```python
from build123d import *

# Parameters (mm, degrees)
BOSS_EXTRUDE1_DEPTH = 5
SKETCH2_W           = 30
SKETCH2_H           = 5
CUT_EXTRUDE1_DEPTH  = 5


with BuildPart() as part:
    # Sketch1 → Boss-Extrude1 (new body)
    with BuildSketch(Plane.XY):
        Polygon((-75.513214474, 35), (-60.513214474, 35), (-60.513214474, 40), (-40.513214474, 40), (-40.513214474, 35), (-25.513214474, 35), (-25.513214474, 40), (-5.513214474, 40), (-5.513214474, 35), (9.486785526, 35), (9.486785526, 40), (29.486785526, 40), (29.486785526, 35), (44.486785526, 35), (44.486785526, 40), (64.486785526, 40), (64.486785526, 35), (79.486785526, 35), (79.486785526, 25), (84.486785526, 25), (84.486785526, 5), (79.486785526, 5), (79.486785526, -5), (84.486785526, -5), (84.486785526, -25), (79.486785526, -25), (79.486785526, -35), (64.486785526, -35), (64.486785526, -40), (44.486785526, -40), (44.486785526, -35), (29.486785526, -35), (29.486785526, -40), (9.486785526, -40), (9.486785526, -35), (-5.513214474, -35), (-5.513214474, -40), (-25.513214474, -40), (-25.513214474, -35), (-40.513214474, -35), (-40.513214474, -40), (-60.513214474, -40), (-60.513214474, -35), (-75.513214474, -35), (-75.513214474, -25), (-80.513214474, -25), (-80.513214474, -5), (-75.513214474, -5), (-75.513214474, 5), (-80.513214474, 5), (-80.513214474, 25), (-75.513214474, 25), align=None)
    extrude(amount=BOSS_EXTRUDE1_DEPTH)

    # Sketch2 → Cut-Extrude1 (cut)
    with BuildSketch(Plane.XY.offset(5)):
        with Locations((39.486785526, -17.5)):
            Rectangle(SKETCH2_W, SKETCH2_H)
        with Locations((-35.513214474, -17.5)):
            Rectangle(SKETCH2_W, SKETCH2_H)
    extrude(amount=-CUT_EXTRUDE1_DEPTH, mode=Mode.SUBTRACT)


solid = part.part
```
Input: part model. Units: mm. Frame: model coordinates. A direction names the side the tool comes from. Coordinates: 2 decimals unless noted, no trailing zeros. Loops run counter-clockwise (first coordinate to the right, second up) from the corner with the lowest first, then second, coordinate; pieces in that order, holes last. Notation, with made-up numbers: M 46.25,83.5 L 87.25,83.5 A14 ccw 87.25,109.5 Z; hole C -4,11 d2. An arc over 180 degrees is marked long. Answer in a Markdown table with one row per item.
1. Section A-A, the plane x = -29.5. Output: boundary loops of the cut face in (y, z).
Response:
| item | result |
|---|---|
| outline | M -35,0 L -20,0 L -20,5 L -35,5 Z; M -15,0 L 35,0 L 35,5 L -15,5 Z |
2. Section B-B, the plane y = -2. Output: boundary loops of the cut face in (x, z), then the cut area to 3 significant figures.
Response:
| item | result |
|---|---|
| outline | M -75.51,0 L 79.49,0 L 79.49,5 L -75.51,5 Z |
| area | 775 mm2 |
3. Section C-C, the plane z = 2.65. Count the separate pieces of the cut face and the enclosed holes in it, then the cut area to 4 significant figures.
Response:
| item | result |
|---|---|
| separate pieces | 1 |
| enclosed holes | 2 |
| area | 11,750 mm2 |
4. Material intervals for line 1 (Y direction, x = -29.5, z = 3.2); line 2 (Y direction, x = 53.5, z = 2.8); line 3 (Y direction, x = 75, z = 4.35), sorted ascending.
Response:
| item | result |
|---|---|
| line 1 | y = -35 to -20, -15 to 35 |
| line 2 | y = -40 to -20, -15 to 40 |
| line 3 | y = -35 to 35 |
5. Reachability of faces 4 (the flat face through (-36, -15, 3)), 5 (the flat face through (2, 35, 2)), 6 (the flat face through (-33, -35, 2)), 7 (the flat face through (-68, -35, 2)) from +Z, -Z, +X, -X, +Y, -Y: full face, straight path, thin tool, end or side. Return the list, or none.
Response:
| item | result |
|---|---|
| face 4 | +Z, -Z |
| face 5 | +Z, -Z, +Y |
| face 6 | +Z, -Z, -Y |
| face 7 | +Z, -Z, -X, -Y |
6. Section D-D, the plane x = 4. Output: boundary loops of the cut face in (y, z), then the cut area to 3 significant figures.
Response:
| item | result |
|---|---|
| outline | M -35,0 L 35,0 L 35,5 L -35,5 Z |
| area | 350 mm2 |
7. First-contact query: pin 1 (2.5 mm diameter, centred on x = -77.5, z = 2, fed in from +Y); pin 2 (1.5 mm diameter, centred on x = 73, z = 1.5, fed in from +Y); pin 3 (2.5 mm diameter, centred on y = 37.5, z = 3, fed in from -X). Flat tips, straight axial feed; report the tip coordinate or a pass-through.
Response:
| item | result |
|---|---|
| pin 1 | stops at y = 25 |
| pin 2 | stops at y = 35 |
| pin 3 | stops at x = -60.51 |
8. Draft query along X for faces 1 (the flat face through (-78, 5, 2)), 2 (the flat face through (79.487, 30, 2)), 3 (the flat face through (-50.513, -18, 3)). Return one class per face: pulls with the +X half, pulls with the -X half, needs draft (parallel to the pull), parting line crosses it, or undercut.
Response:
| item | result |
|---|---|
| face 1 | needs draft |
| face 2 | pulls with the +X half |
| face 3 | undercut |
